from build123d import *

# Parameters (mm, degrees)
SKETCH1_R           = 3.175
SKETCH1_R_2         = 2.54
BOSS_EXTRUDE1_DEPTH = 12.7
BOSS_EXTRUDE2_DEPTH = 2.54


with BuildPart() as part:
    # Sketch1 → Boss-Extrude1 (new body)
    with BuildSketch(Plane(origin=(0, 0, 0), x_dir=(1, 0, 0), z_dir=(0, 1, 0))):
        with Locations(Location((0, 0, 0), (0, 0, 270))):
            Circle(SKETCH1_R)
        with Locations(Location((0, 0, 0), (0, 0, 270))):
            Circle(SKETCH1_R_2, mode=Mode.SUBTRACT)
    extrude(amount=BOSS_EXTRUDE1_DEPTH)

    # Sketch3 → Boss-Extrude2 (add)
    with BuildSketch(Plane(origin=(0, 12.7, 0), x_dir=(1, 0, 0), z_dir=(0, 1, 0))):
        with BuildLine():
            Line((-1.27, 4.259709497), (-1.27, 2.909935566))
            ThreePointArc((-1.27, 2.909935566), (0, -3.175), (1.27, 2.909935566))
            Line((1.27, 2.909935566), (1.27, 4.259709497))
            ThreePointArc((1.27, 4.259709497), (0, 4.445), (-1.27, 4.259709497))
        make_face()
    extrude(amount=BOSS_EXTRUDE2_DEPTH)


solid = part.part
CAD build for the part. Positions are in the model's coordinates, mm. A direction names the side the tool comes from. Give positions to 0.01 mm unless a question says otherwise; leave off trailing zeros. Order: outer loops, then holes, each group sorted by start corner. A loop starts at its lowest first (then second) coordinate and runs counter-clockwise, first axis right, second up. Notation, with made-up numbers: (35, 6.5) -> (54, 6.5) arc R11 cw to (54, 25.5) -> close; hole circle Ø10 at (26.5, -18.5). An arc over 180 degrees is marked (long way). Return JSON: item names as keys, results as strings.
Q1. Which spindle directions (+Z, -Z, +X, -X, +Y, -Y) get a long thin tool onto all of the face, cutting with end or side? Do faces 1 (the face through (0.018, 13.952, -4.445)), 2 (the face through (1.27, 14, -4)). Say none if no direction does.
Working result:
{"face 1": "-Z, +Y, -Y", "face 2": "-Z, +X, +Y, -Y"}
Q2. Drill centre lines: line 1 (X direction, y = 2.75, z = 0) (3 decimals); line 2 (Y direction, x = -2.5, z = 0); line 3 (Z direction, x = -1.25, y = 11). Where is each one in solid material? Low to high.
Working result:
{"line 1": "-3.175 to -2.54, 2.54 to 3.175", "line 2": "12.7 to 15.24", "line 3": "-2.92 to -2.21, 2.21 to 2.92"}
Q3. Saw through at C-C (y = 5.75). Write the cut outline in (x, z) (3 decimals), then the cut area to 3 significant figures.
Working result:
{"outline": "circle Ø6.35 at (0, 0); hole circle Ø5.08 at (0, 0)", "area": "11.4 mm²"}
Q4. Saw through at D-D (z = -2). Write the cut outline in (x, y).
Working result:
{"outline": "(-2.47, 0) -> (-1.57, 0) -> (-1.57, 12.7) -> (1.57, 12.7) -> (1.57, 0) -> (2.47, 0) -> (2.47, 15.24) -> (-2.47, 15.24) -> close"}
Q5. Saw through at B-B (x = 0). Write the cut outline in (y, z) (3 decimals), then the cut area to 3 significant figures.
Working result:
{"outline": "(0, -3.175) -> (12.7, -3.175) -> (12.7, -4.445) -> (15.24, -4.445) -> (15.24, 3.175) -> (0, 3.175) -> (0, 2.54) -> (12.7, 2.54) -> (12.7, -2.54) -> (0, -2.54) -> close", "area": "35.5 mm²"}
Q6. Saw through at A-A (z = 0). Write the cut outline in (x, y) (3 decimals).
Working result:
{"outline": "(-3.175, 0) -> (-2.54, 0) -> (-2.54, 12.7) -> (2.54, 12.7) -> (2.54, 0) -> (3.175, 0) -> (3.175, 15.24) -> (-3.175, 15.24) -> close"}
Q7. Flat gauge pins, fed straight in: pin 1 (3 mm diameter, centred on x = 0, z = 0, fed in from -Y); pin 2 (0.7 mm diameter, centred on y = 14.5, z = -3.5, fed in from -X); pin 3 (1.1 mm diameter, centred on y = 14.5, z = -3.5, fed in from +X). Where does each tip first touch, or does it go through?
Working result:
{"pin 1": "y = 12.7", "pin 2": "x = -1.27", "pin 3": "x = 1.27"}
Q8. Mould opens along X. For faces 3 (the face through (-1.27, 14, -4)), 4 (the face through (2.52, 6.26, -0.33)), 5 (the face through (0, 12.7, 0)), 6 (the face through (0, 15.24, -1)) say: pulls with the +X half, pulls with the -X half, needs draft (parallel to the pull), parting line crosses it, or undercut.
Working result:
{"face 3": "pulls with the -X half", "face 4": "undercut", "face 5": "undercut", "face 6": "needs draft"}
